Autodesk Inventor part; units mm, degrees
ref_plane "Work Plane1" through (0, -2.75, 0) normal (0, -1, 0) x (1, 0, 0)
ref_plane "YZ Plane" through (0, 0, 0) normal (1, 0, 0) x (0, 1, 0)
ref_plane "XZ Plane" through (0, 0, 0) normal (0, 1, 0) x (-1, 0, 0)
sketch "Sketch1" plane through (0, 0, 0) normal (0, 1, 0) x (-1, 0, 0)
  line L0 (0, 0) -> (200, 0)
  line L1 (200, 0) -> (200, -80)
  line L2 (200, -80) -> (0, -80)
  line L3 (0, -80) -> (0, 0)
  line L4 (10, -30) -> (30, -30)
  line L5 (30, -30) -> (30, -50)
  line L6 (30, -50) -> (10, -50)
  line L7 (10, -50) -> (10, -30)
  circle A0 centre (10, -30) radius 1.5
  circle A1 centre (30, -50) radius 1.5
  circle A2 centre (30, -30) radius 1.5
  circle A3 centre (10, -50) radius 1.5
  line L8 (192.5, -7.5) -> (162.5, -7.5)
  line L9 (162.5, -7.5) -> (162.5, -72.5)
  line L10 (162.5, -72.5) -> (192.5, -72.5)
  line L11 (192.5, -72.5) -> (192.5, -7.5)
  circle A4 centre (192.5, -7.5) radius 1.5
  circle A5 centre (192.5, -72.5) radius 1.5
  circle A6 centre (162.5, -72.5) radius 1.5
  circle A7 centre (162.5, -7.5) radius 1.5
  line L12 (200, 0) -> (152.5, 0)
  line L13 (152.5, 0) -> (152.5, -80)
  line L14 (152.5, -80) -> (200, -80)
  line L15 (200, -80) -> (200, 0)
  line L16 (152.5, -20) -> (0, -20)
  line L17 (0, -20) -> (0, -60)
  line L18 (0, -60) -> (152.5, -60)
  line L19 (152.5, -60) -> (152.5, -20)
  line L20 (40, -20) -> (40, -60)
  point P0 (191, -7.5)
  point P1 (192.5, -9)
  point P2 (192.5, -71)
  point P3 (191, -72.5)
  point P4 (164, -72.5)
  point P5 (162.5, -71)
  point P6 (164, -7.5)
  point P7 (162.5, -9)
  point P8 (152.5, 0)
  point P9 (0, -20)
  dimension "d0" = 200
  dimension "d1" = 80
  dimension "d2" = 20
  dimension "d3" = 20
  dimension "d4" = 30
  dimension "d5" = 10
  dimension "d6" = 3
  dimension "d7" = 3
  dimension "d8" = 3
  dimension "d9" = 3
  dimension "d10" = 65
  dimension "d11" = 30
  dimension "d12" = 7.5
  dimension "d13" = 7.5
  dimension "d14" = 3
  dimension "d15" = 3
  dimension "d16" = 3
  dimension "d17" = 3
  dimension "d18" = 20
  dimension "d19" = 20
  dimension "d20" = 10
  dimension "d23" = 40
extrude "Extrusion1" add sketch "Sketch1" along normal blind 3 contours L0 L1 L2 L13 | L16 L20 L18 L3 | L13 L18 L20 L16 | L4 A2 L5 A1 L6 A3 L7 A0 | L8 A4 L11 A5 L10 A6 L9 A7
extrude "Extrusion2" add sketch "Sketch1" against normal blind 5.5 contours L0 L1 L2 L13 | L13 L18 L20 L16 | L8 A4 L11 A5 L10 A6 L9 A7
ref_plane "Work Plane1" through (0, -2.75, 0) normal (0, -1, 0) x (1, 0, 0)
mirror "Mirror1" about plane through (0, -2.75, 0) normal (0, -1, 0) of "Extrusion1"
chamfer "Chamfer1" distance 12.5 angle 45 4 edges at (0, 1.5, -20) (0, -7, -20) (0, -7, -60) (0, 1.5, -60)
sketch "Sketch3" plane through (-152.5, -8.5, -20) normal (0, 0, 1) x (1, 0, 0)
  line L0 (152.5, 11.5) -> (0, 11.5)
  line L1 (140, 11.5) -> (40, 11.5)
  line L2 (40, 11.5) -> (40, -40)
  line L3 (40, -40) -> (140, -40)
  line L4 (140, -40) -> (140, 11.5)
  line L5 (112.5, 8.5) -> (112.5, 3)
  line L6 (112.5, 3) -> (140, 3)
  line L7 (112.5, 8.5) -> (112.5, 3)
  line L8 (112.5, 8.5) -> (140, 8.5)
  line L9 (0, 11.5) -> (140, 11.5)
  line L10 (0, 0) -> (0, 11.5)
  line L11 (0, 0) -> (140, 0)
  line L12 (0, 0) -> (140, 0)
  line L13 (122.5, 0) -> (122.5, 11.5)
  line L14 (0, 11.5) -> (152.5, 11.5)
  line L15 (140, -40) -> (140, -32.5)
  circle A0 centre (134.5, -32.5) radius 1.5
  line L16 (140, -32.5) -> (40, -32.5)
  circle A1 centre (45, -32.5) radius 1.5
  line L17 (140, 3) -> (140, 0)
  line L18 (140, 11.5) -> (140, 8.5)
  point P0 (152.5, 8.5)
  point P1 (147.5, 11.5)
  point P2 (140, 3)
  point P3 (140, 8.5)
  point P4 (40, 11.5)
  dimension "d30" = 100
  dimension "d32" = 7.5
  dimension "d33" = 3
  dimension "d34" = 3
  dimension "d35" = 89.5
  dimension "d36" = 5
  dimension "d40" = 40
extrude "Extrusion3" add sketch "Sketch3" along normal blind 6 contours L4 L8 L13 L0 | L13 L8 L5 L6 L11 L2 L0 | L4 L11 L13 L6 | L11 L4 L16 A0 A1 L2 | L16 A1 A0 L4 L3 L2
sketch "Sketch4" plane through (-152.5, -8.5, -20) normal (0, 0, -1) x (-1, 0, 0)
  line L0 (-40, 11.5) -> (-40, -40)
  line L1 (-40, 0) -> (-140, 0)
  line L2 (-140, 0) -> (-140, -6)
  line L3 (-140, -6) -> (-40, -6)
  line L4 (-40, -6) -> (-40, 0)
  line L5 (-140, -40) -> (-140, 0)
  line L6 (-90, -6) -> (-90, 0)
  line L7 (-140, 0) -> (0, 0)
  point P0 (-152.5, 8.5)
  point P1 (-162.5, 0)
  dimension "d39" = 6
extrude "Extrusion4" add sketch "Sketch4" along normal blind 30 contours L0 L3 L6 L1
fillet "Fillet2" radius 10 4 edges at (-200, -2.75, -80) (-152.5, -2.75, -80) (-152.5, -2.75, 0) (-200, -2.75, 0)
properties part number "RobotBaseMotorExt"
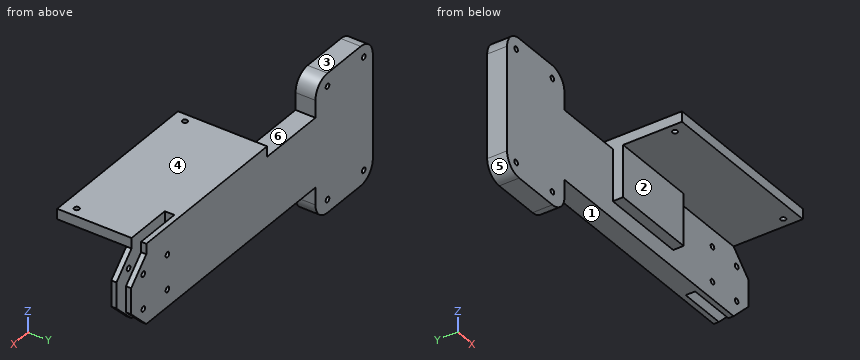
Work out the finished part from the listing and answer in its coordinate system (mm). Face numbers are marked on the shaded views. A direction names the side the tool comes from. Give positions to 0.01 mm unless a question says otherwise; leave off trailing zeros. Loops run counter-clockwise (first coordinate to the right, second up) from the corner with the lowest first, then second, coordinate; pieces in that order, holes last. Notation, with made-up numbers: (-18, -20) -> (27, -20) arc R21 cw to (27, 17) -> close; hole circle Ø6 at (1.5, 63). An arc over 180 degrees is marked (long way). Write item = value, one per line. Start each with the question number.
(1) Find section B-B on x = -181. Give the vertices of the cut face in (y, z), and give its area (3 significant figures).
(2) Find section A-A on y = -28. Give the vertices of the cut face in (x, z).
(3) Given pin 1 Ø1.8 at (x, z) = (-162.5, -72.5) entering from +Y; pin 2 Ø18 at (y, z) = (-11.5, -27) entering from -X; pin 3 Ø5 at (x, y) = (-106, -13.5) entering from -Z; pin 4 Ø2.5 at (y, z) = (2, -18) entering from +X, each flat-ended and moving along its own axis, determine where each tip first touches the part or whether it passes through.
(4) Find the intervals of material crossed by probe 1 along Y at (x, z) = (-33.5, -41.5); probe 2 along X at (y, z) = (-1, -7); probe 3 along X at (y, z) = (-7.25, -30), in increasing order. Write a range as from..to.
(5) Which of the six approach directions +Z, -Z, +X, -X, +Y, -Y give full straight-line access (tool end or side, diameter ignored) to the marked faces 1, 2 and 3?
(6) The mould has two halves that part along X. Classify the marked faces 4, 5 and 6: +X half, -X half, draft (parallel to the pull), parting line (faces both ways), or undercut.
From the geometry:
q1.outline = (-8.5, -80) -> (3, -80) -> (3, 0) -> (-8.5, 0) -> close
q1.area = 920 mm^2
q2.outline = (-112.5, -20) -> (-12.5, -20) -> (-12.5, -14) -> (-112.5, -14) -> close
q3.pin_1 = through
q3.pin_2 = -200
q3.pin_3 = -50
q3.pin_4 = -12.5
q4.probe_1 = -8.5..-5.5, 0..3
q4.probe_2 = -199.54..-193.91, -191.09..-163.91, -161.09..-152.96
q4.probe_3 = -200..-31.5, -28.5..-11.5, -8.5..-2.5
q5.face_1 = -Z, +X, +Y, -Y
q5.face_2 = -Z, +X, -X, -Y
q5.face_3 = +Z, +X, -X, +Y, -Y
q6.face_4 = draft
q6.face_5 = -X half
q6.face_6 = undercut
